Can you work these out from the model? Positions are in its coordinate system, mm. A direction names the side the tool comes from. Coordinates: 2 decimals unless noted, no trailing zeros. Loops run counter-clockwise (first coordinate to the right, second up) from the corner with the lowest first, then second, coordinate; pieces in that order, holes last.
```python
from build123d import *

# Parameters (mm, degrees)
F1_DEPTH = 50
F2_R     = 5
F3_T     = -2.5


with BuildPart() as f1:
    # F0 (on Front) → F1 (new body, symmetric)
    with BuildSketch(Plane.XZ):
        Polygon((0, 20), (0, 0), (20, 0), (20, 5), (5, 5), (5, 20), align=None)
    extrude(amount=F1_DEPTH, both=True)

    # F2
    f2_edges = [f1.edges().sort_by_distance(p)[0] for p in [
        (2.5, -50, 20),
        (2.5, 50, 20),
        (20, -50, 2.5),
        (20, 50, 2.5),
    ]]
    fillet(f2_edges, radius=F2_R)

    # F3
    f3_openings = [f1.faces().sort_by_distance(p)[0] for p in [
        (12.45401, 0, 5),
        (5, 0, 12.45401),
    ]]
    offset(amount=F3_T, openings=f3_openings)


solid = f1.part
```
(1) If I drill on probe 1 along Y at (x, z) = (4.25, 9); probe 2 along X at (y, z) = (-38, 3.5), over which ranges is the centre line in solid material (lowest first)?
Check values:
probe 1: y = -50 to -47.5, 47.5 to 50
probe 2: x = 0 to 2.5, 17.5 to 20
(2) I want a section at C-C on x = 9.5. Write out the boundary of the cut face in (y, z).
Check values:
outline: (-50, 0) - (50, 0) - (50, 5) - (47.5, 5) - (47.5, 2.5) - (-47.5, 2.5) - (-47.5, 5) - (-50, 5) - close
(3) I want a section at D-D on z = 12.5. Write out the boundary of the cut face in (x, y), then the cut area to 4 significant figures.
Check values:
outline: (0, -50) - (5, -50) - (5, -47.5) - (2.5, -47.5) - (2.5, 47.5) - (5, 47.5) - (5, 50) - (0, 50) - close
area: 262.5 mm2
(4) I want a section at B-B on y = 32. Write out the boundary of the cut face in (x, z), then the cut area to 3 significant figures.
Check values:
outline: (0, 0) - (20, 0) - (20, 5) - (17.5, 5) - (17.5, 2.5) - (2.5, 2.5) - (2.5, 17.5) - (5, 17.5) - (5, 20) - (0, 20) - close
area: 106 mm2
(5) I'm going to push flat-ended pins straight in: pin 1 (2 mm diameter, centred on y = 7.5, z = 13.5, fed in from +X); pin 2 (2 mm diameter, centred on x = 4, y = 18, fed in from -Z); pin 3 (4.5 mm diameter, centred on x = 10, y = 15.5, fed in from +Z). Where does each tip first touch, or does it pass through?
Check values:
pin 1: stops at x = 2.5
pin 2: stops at z = 0
pin 3: stops at z = 2.5
(6) Which directions (+Z, -Z, +X, -X, +Y, -Y) give clear straight access to the entire face, cutting with the end or side of a thin tool? Please do faces 5 (the flat face through (5.9, -47.5, 4.7)), 6 (the cylindrical face through (16.787, 46.748, 3.768)), 7 (the flat face through (4, -1, 17.5)), 8 (the flat face through (5, 0, 19)).
Check values:
face 5: none
face 6: +Z
face 7: +X
face 8: +Z, +X, +Y, -Y
(7) I want a section at A-A on x = 3.75. Write out the boundary of the cut face in (y, z), then the cut area to 3 significant figures.
Check values:
outline: (-50, 0) - (50, 0) - (50, 15) arc R5 ccw to (45, 20) - (-45, 20) arc R5 ccw to (-50, 15) - close; hole (-47.5, 2.5) - (47.5, 2.5) - (47.5, 15) arc R2.5 ccw to (45, 17.5) - (-45, 17.5) arc R2.5 ccw to (-47.5, 15) - close
area: 567 mm2
(8) If we mould it in two halves opening along Y, with no side actions, what happens to faces 1 (the cylindrical face through (2, 48, 19)), 2 (the cylindrical face through (3.732, -46.748, 16.787)), 3 (the flat face through (3, -1, 20)), 4 (the flat face through (17.5, -1, 4))? For each: released by +Y, released by -Y, zero draft, split by the parting line, or undercut.
Check values:
face 1: released by +Y
face 2: undercut
face 3: zero draft
face 4: undercut
